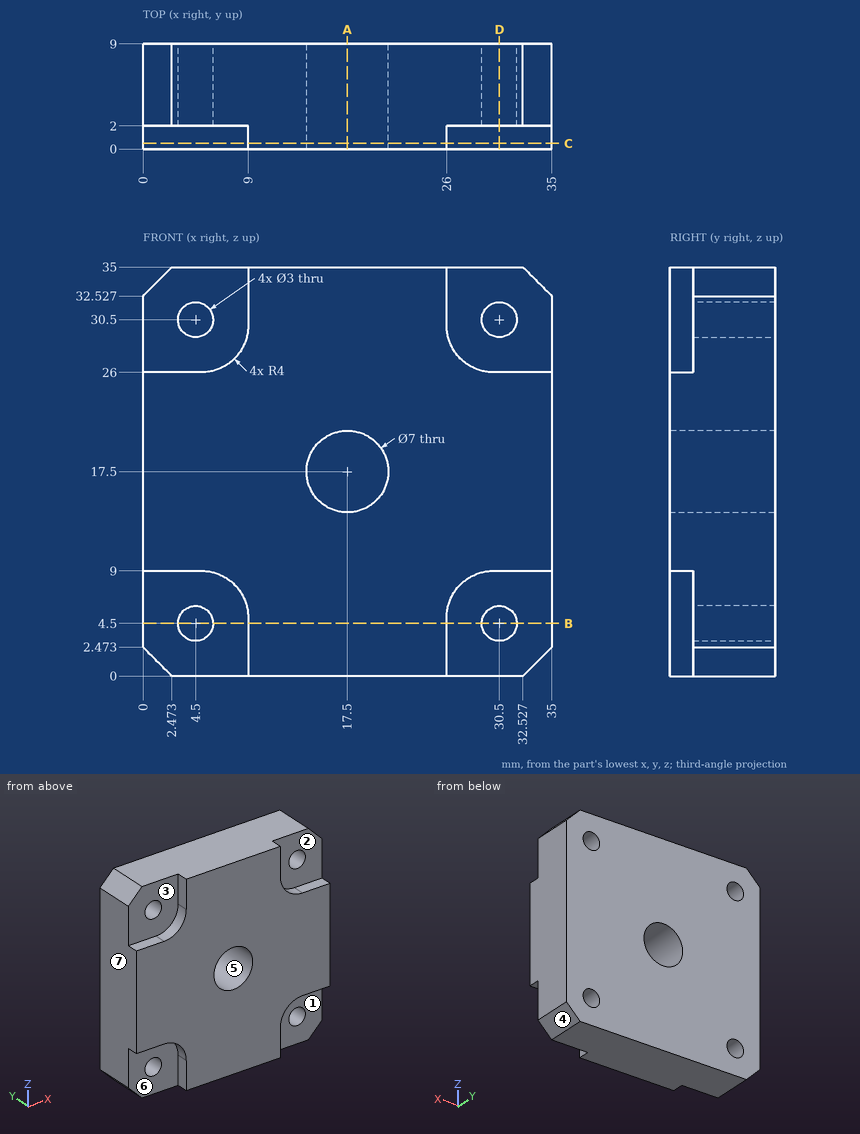
For this review, use the dimensioned drawing (mm, ordinates from the lowest corner) and the shaded views. A direction names the side the tool comes from. Give positions to 0.01 mm unless a question says otherwise; leave off trailing zeros. Order: outer loops, then holes, each group sorted by start corner. A loop starts at its lowest first (then second) coordinate and runs counter-clockwise, first axis right, second up. Notation, with made-up numbers: (60.5, -37.75) - (90.5, -37.75) arc R33 ccw to (90.5, 1.25) - close; hole circle Ø7 at (40, 35). An arc over 180 degrees is marked (long way). Use a Markdown table: item, result. Add a question column.
(1) Add section A-A on x = 17.5. Give the boundary of the cut face in (y, z).
(2) Add section B-B on z = 4.5. Give the boundary of the cut face in (x, y).
(3) Wall thickness on probe 1 along X at (y, z) = (6.25, 4.5); probe 2 along X at (y, z) = (5.25, 17.5); probe 3 along Z at (x, y) = (31, 3): over which ranges is each line inside the solid? List them lowest first. Write a range as [from, to].
(4) Add section D-D on x = 30.5. Give the boundary of the cut face in (y, z), then the cut area to 3 significant figures.
(5) Clearance check with flat-ended pins moving along their axes: P1, Ø1.6, axis at y = 0.5, z = 1.5, coming from the -X side; P2, Ø1.6, axis at x = 32, y = 1, coming from the -Z side; P3, Ø3.5, axis at x = 30.5, z = 30.5, coming from the -Y side. State where each tip first meets the part, or that it passes through.
(6) Mouldability with a two-part tool opening along X and no side actions: class the marked faces 4, 5, 6 and 7 as +X half, -X half, draft (parallel to the pull), parting line (faces both ways), or undercut.
(7) Add section C-C on y = 0.5. Give the boundary of the cut face in (x, z), then the cut area to 3 significant figures.
(8) Machinability: for the marked faces 1, 2 and 3, which of the approach directions +Z, -Z, +X, -X, +Y, -Y give a long, thin tool a straight path to every point of the face, cutting with its end or side? Answer none if there is none.
Report:
| question | item | result |
|---|---|---|
| 1 | outline | (0, 0) - (9, 0) - (9, 14) - (0, 14) - close; (0, 21) - (9, 21) - (9, 35) - (0, 35) - close |
| 2 | outline | (0, 2) - (3, 2) - (3, 9) - (0, 9) - close; (6, 2) - (9, 2) - (9, 0) - (26, 0) - (26, 2) - (29, 2) - (29, 9) - (6, 9) - close; (32, 2) - (35, 2) - (35, 9) - (32, 9) - close |
| 3 | probe 1 | x = [0, 3], [6, 29], [32, 35] |
| 3 | probe 2 | x = [0, 14], [21, 35] |
| 3 | probe 3 | z = [0, 3.09], [5.91, 29.09], [31.91, 35] |
| 4 | outline | (0, 9) - (2, 9) - (2, 6) - (9, 6) - (9, 29) - (2, 29) - (2, 26) - (0, 26) - close; (2, 0) - (9, 0) - (9, 3) - (2, 3) - close; (2, 32) - (9, 32) - (9, 35) - (2, 35) - close |
| 4 | area | 237 mm² |
| 5 | P1 | stops at x = 9 |
| 5 | P2 | stops at z = 9 |
| 5 | P3 | stops at y = 2 |
| 6 | face 4 | +X half |
| 6 | face 5 | undercut |
| 6 | face 6 | draft |
| 6 | face 7 | -X half |
| 7 | outline | (0, 9) - (5, 9) arc R4 cw to (9, 5) - (9, 0) - (26, 0) - (26, 5) arc R4 cw to (30, 9) - (35, 9) - (35, 26) - (30, 26) arc R4 cw to (26, 30) - (26, 35) - (9, 35) - (9, 30) arc R4 cw to (5, 26) - (0, 26) - close; hole circle Ø7 at (17.5, 17.5) |
| 7 | area | 876 mm² |
| 8 | face 1 | -Z, +X, -Y |
| 8 | face 2 | +Z, +X, -Y |
| 8 | face 3 | +Z, -X, -Y |
